Here's how the part is built. I have some questions about the finished solid (model axes, mm). Give positions to 0.01 mm unless a question says otherwise; leave off trailing zeros. Write each loop counter-clockwise with the first axis right and the second up, starting at its lowest first coordinate (ties: lowest second). Pieces come first, ordered by that corner, then holes. Notation, with made-up numbers: (40, 87.25) -> (97, 87.25) arc R15 cw to (97, 114.25) -> close; hole circle Ø1 at (-12.75, 3.5). An arc over 180 degrees is marked (long way). Use CSV: the item, a comma, the result in double quotes. Start each with the question number.
(1) Suppose I cut it at D-D on y = 11.75. List the corners of the cut face in (x, z) for me.
(2) Suppose I cut it at B-B on x = 0. List the corners of the cut face in (y, z) for me, plus the area to 3 significant figures.
(3) If we mould it in two halves opening along X, with no side actions, what happens to faces 1 (the cylindrical face through (14.246, 22.345, 0.74)), 2 (the cylindrical face through (-22, -11.7, 0.8)), 3 (the flat face through (-6, 20, 0))? For each: pulls with the +X half, pulls with the -X half, needs draft (parallel to the pull), parting line crosses it, or undercut.
(4) Suppose I cut it at C-C on x = -11.5. List the corners of the cut face in (y, z) for me, plus the area to 3 significant figures.
(5) For pin 1 Ø3 at (x, y) = (-20.35, 11.75) entering from -Z, with a flat end and sliding along its axis, tell me the tip position at first contact or that it passes through.
(6) I need wall thicknesses on L1, parallel to Y at x = 0, z = 0.9; L2, parallel to Y at x = 1, z = 0.5; L3, parallel to X at y = 6.5, z = 0.85. Which ranges of each line are inside material? Lowest first, please. Write a range as [from, to].
(7) Suppose I cut it at A-A on y = 0. List the corners of the cut face in (x, z) for me, plus the area to 3 significant figures.
from build123d import *

# Parameters (mm, degrees)
SKETCH_1_R               = 26.5
SKETCH_1_R_2             = 20.5
EXTRUDE_1_DEPTH          = 1.5
SKETCH_2_R               = 1.65
CUT_EXTRUDE_1_DEPTH      = 1.5
PATTERN_CIRCULAR_1_COUNT = 6


with BuildPart() as part:
    # 草图1 → 凸台-拉伸1 (new body)
    with BuildSketch(Plane.XY):
        Circle(SKETCH_1_R)
        Circle(SKETCH_1_R_2, mode=Mode.SUBTRACT)
    extrude(amount=EXTRUDE_1_DEPTH)

    # 草图2 → 切除-拉伸1 (cut)
    with BuildSketch(Plane.XY.offset(1.5)):
        with Locations((0, 23.5)):
            Circle(SKETCH_2_R)
    cut_extrude_1 = extrude(amount=-CUT_EXTRUDE_1_DEPTH, mode=Mode.SUBTRACT)

    # 阵列(圆周)1: 切除-拉伸1 ×6 about axis
    pattern_circular_1_axis = Axis((0, 0, 0), (0, 0, 1))
    for i in range(1, PATTERN_CIRCULAR_1_COUNT):
        add(cut_extrude_1.rotate(pattern_circular_1_axis, i * 360 / PATTERN_CIRCULAR_1_COUNT), mode=Mode.SUBTRACT)


solid = part.part
Geometry says:
1,outline,"(-23.75, 0) -> (-22, 0) -> (-22, 1.5) -> (-23.75, 1.5) -> close; (-18.7, 0) -> (-16.8, 0) -> (-16.8, 1.5) -> (-18.7, 1.5) -> close; (16.8, 0) -> (18.7, 0) -> (18.7, 1.5) -> (16.8, 1.5) -> close; (22, 0) -> (23.75, 0) -> (23.75, 1.5) -> (22, 1.5) -> close"
2,outline,"(-26.5, 0) -> (-25.15, 0) -> (-25.15, 1.5) -> (-26.5, 1.5) -> close; (-21.85, 0) -> (-20.5, 0) -> (-20.5, 1.5) -> (-21.85, 1.5) -> close; (20.5, 0) -> (21.85, 0) -> (21.85, 1.5) -> (20.5, 1.5) -> close; (25.15, 0) -> (26.5, 0) -> (26.5, 1.5) -> (25.15, 1.5) -> close"
2,area,"8.10 mm²"
3,face 1,"parting line crosses it"
3,face 2,"undercut"
3,face 3,"needs draft"
4,outline,"(-23.87, 0) -> (-16.97, 0) -> (-16.97, 1.5) -> (-23.87, 1.5) -> close; (16.97, 0) -> (23.87, 0) -> (23.87, 1.5) -> (16.97, 1.5) -> close"
4,area,"20.7 mm²"
5,pin 1,"through"
6,L1,"[-26.5, -25.15], [-21.85, -20.5], [20.5, 21.85], [25.15, 26.5]"
6,L2,"[-26.48, -24.81], [-22.19, -20.48], [20.48, 22.19], [24.81, 26.48]"
6,L3,"[-25.69, -19.44], [19.44, 25.69]"
7,outline,"(-26.5, 0) -> (-20.5, 0) -> (-20.5, 1.5) -> (-26.5, 1.5) -> close; (20.5, 0) -> (26.5, 0) -> (26.5, 1.5) -> (20.5, 1.5) -> close"
7,area,"18.0 mm²"
